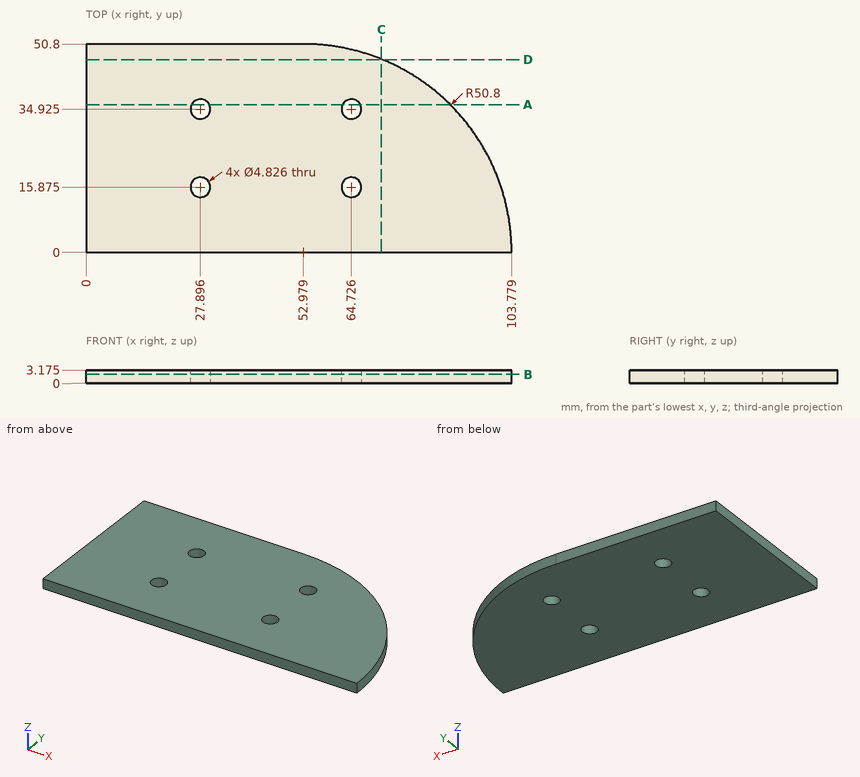
Verification items for this drawing (mm, ordinates from the low corner). Round coordinates to 2 decimals unless told otherwise and drop trailing zeros. Loops run counter-clockwise (first coordinate to the right, second up) from the corner with the lowest first, then second, coordinate; pieces in that order, holes last. Notation, with made-up numbers: (-29.75, 51.25) -> (20.25, 51.25) arc R9 ccw to (20.25, 62.25) -> close; hole circle Ø8 at (47, -1). An arc over 180 degrees is marked (long way). Write item = value, one per line. Start each with the question number.
1) Sectioned sample at B-B, the plane z = 2.2. Record the cut outline in (x, y) (1 decimal), plus the area to 4 significant figures.
2) Sectioned sample at D-D, the plane y = 47. Record the cut outline in (x, z) (1 decimal).
3) Thickness scan on probe 1 along X at (y, z) = (36, 1.15) (1 decimal); probe 2 along X at (y, z) = (17.5, 1.05) (1 decimal); probe 3 along Y at (x, z) = (65, 0.25). Record the ranges inside material, lowest first.
4) Sectioned sample at C-C, the plane x = 72. Record the cut outline in (y, z) (1 decimal).
5) Sectioned sample at A-A, the plane y = 36. Record the cut outline in (x, z) (1 decimal).
6) Gauge pin test, flat end, axial feed: pin 1 Ø1.5 at (x, z) = (77.5, 1) entering from -Y. Record the tip position at first contact, or that the pin passes through.
Results are:
q1.outline = (0, 0) -> (103.8, 0) arc R50.8 ccw to (53, 50.8) -> (0, 50.8) -> close; hole circle Ø4.8 at (27.9, 15.9); hole circle Ø4.8 at (27.9, 34.9); hole circle Ø4.8 at (64.7, 15.9); hole circle Ø4.8 at (64.7, 34.9)
q1.area = 4,645 mm^2
q2.outline = (0, 0) -> (72.3, 0) -> (72.3, 3.2) -> (0, 3.2) -> close
q3.probe_1 = 0 to 25.7, 30.1 to 62.6, 66.9 to 88.8
q3.probe_2 = 0 to 26.1, 29.7 to 62.9, 66.5 to 100.7
q3.probe_3 = 0 to 13.48, 18.27 to 32.53, 37.32 to 49.36
q4.outline = (0, 0) -> (47.1, 0) -> (47.1, 3.2) -> (0, 3.2) -> close
q5.outline = (0, 0) -> (25.7, 0) -> (25.7, 3.2) -> (0, 3.2) -> close; (30.1, 0) -> (62.6, 0) -> (62.6, 3.2) -> (30.1, 3.2) -> close; (66.9, 0) -> (88.8, 0) -> (88.8, 3.2) -> (66.9, 3.2) -> close
q6.pin_1 = 0
